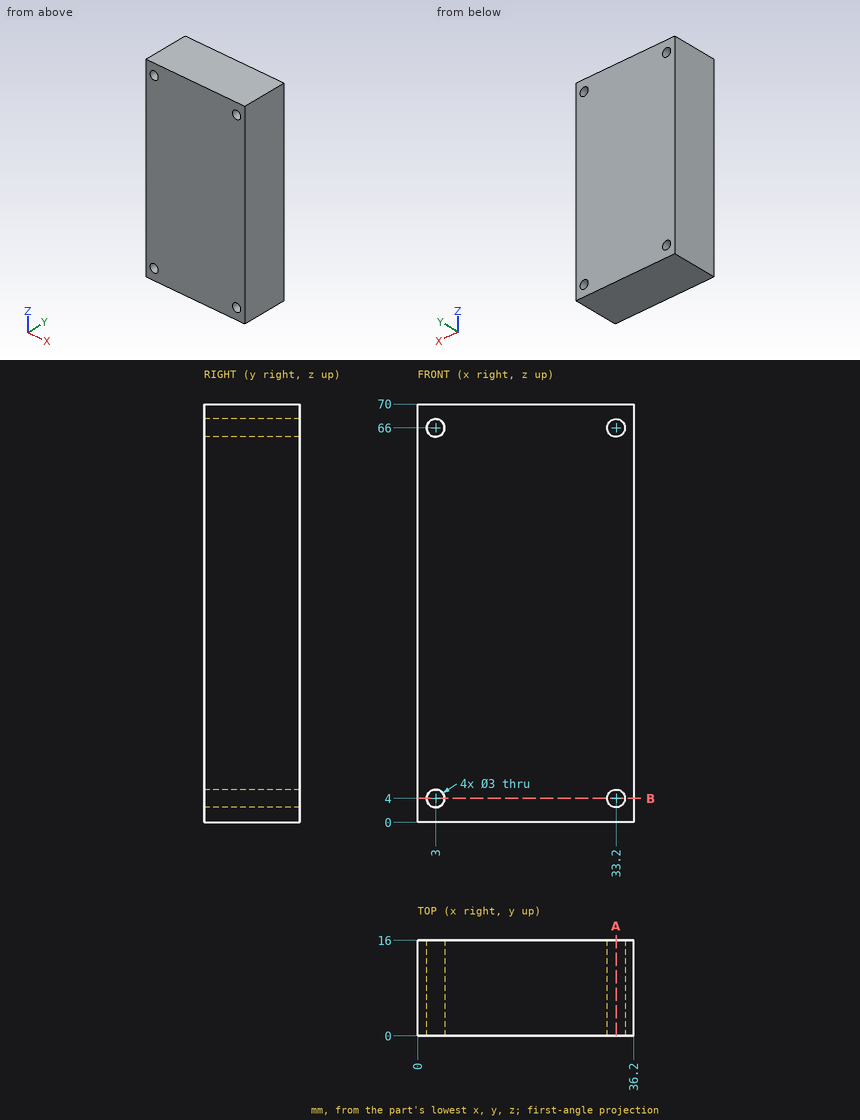
Drawing for the job (mm, zero at the part's lowest x, y, z). Give positions to 0.01 mm unless a question says otherwise; leave off trailing zeros. Loops run counter-clockwise (first coordinate to the right, second up) from the corner with the lowest first, then second, coordinate; pieces in that order, holes last.
Item 1: Drill centre lines: line 1 along Z through (x, y) = (3, 12); line 2 along X through (y, z) = (5, 66). Where is each one in solid material? Low to high.
Check values:
line 1: z = 0 to 2.5, 5.5 to 64.5, 67.5 to 70
line 2: x = 0 to 1.5, 4.5 to 31.7, 34.7 to 36.2
Item 2: Slice it at A-A (x = 33.2). Write the cut outline in (y, z), plus the area to 3 significant figures.
Check values:
outline: (0, 0) - (16, 0) - (16, 2.5) - (0, 2.5) - close; (0, 5.5) - (16, 5.5) - (16, 64.5) - (0, 64.5) - close; (0, 67.5) - (16, 67.5) - (16, 70) - (0, 70) - close
area: 1,020 mm2
Item 3: Slice it at B-B (z = 4). Write the cut outline in (x, y).
Check values:
outline: (0, 0) - (1.5, 0) - (1.5, 16) - (0, 16) - close; (4.5, 0) - (31.7, 0) - (31.7, 16) - (4.5, 16) - close; (34.7, 0) - (36.2, 0) - (36.2, 16) - (34.7, 16) - close
